Print and shaded views of the part. All mm, measured from the part's lowest x, y and z. Coordinates: 2 decimals unless noted, no trailing zeros. Order: outer loops, then holes, each group sorted by start corner. A loop starts at its lowest first (then second) coordinate and runs counter-clockwise, first axis right, second up.
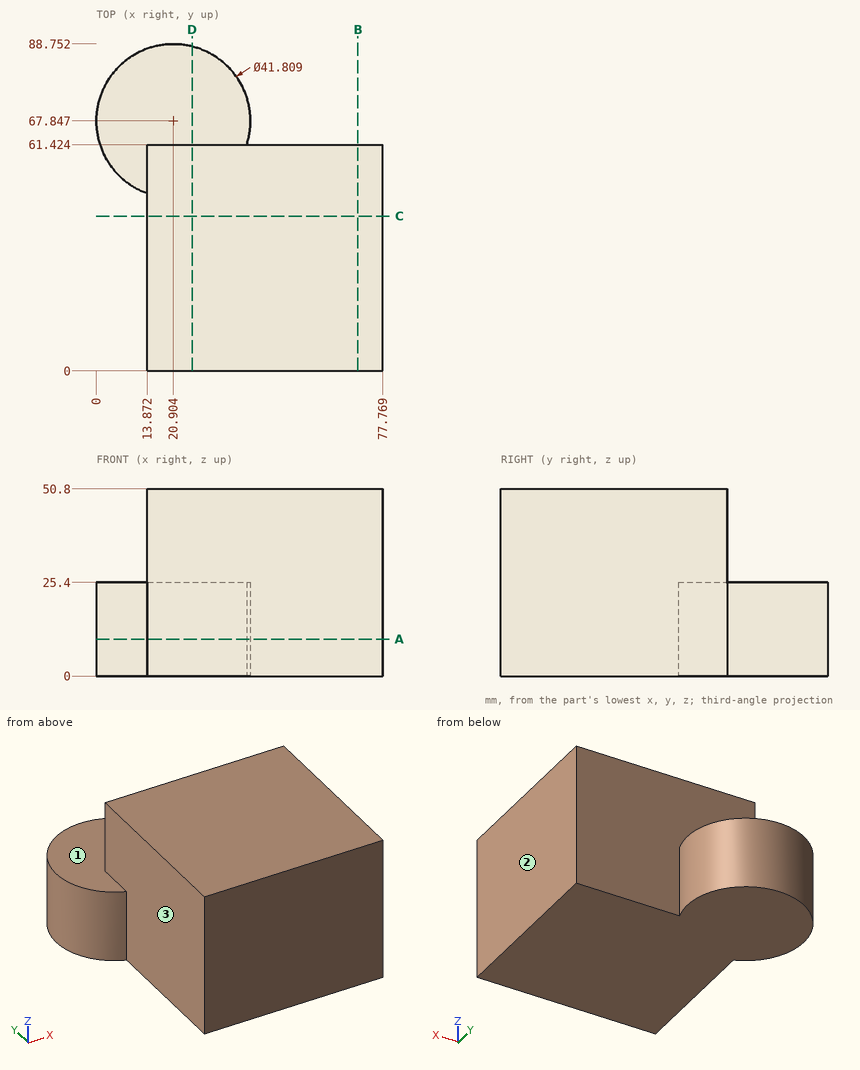
Q1. Cut at A-A, the plane z = 10. List the corners of the cut face in (x, y) (1 decimal).
Established:
outline: (13.9, 0) - (77.8, 0) - (77.8, 61.4) - (40.8, 61.4) arc R20.9 ccw (long way) to (13.9, 48.2) - close
Q2. Cut at D-D, the plane x = 26. List the corners of the cut face in (y, z) (1 decimal).
Established:
outline: (0, 0) - (88.1, 0) - (88.1, 25.4) - (61.4, 25.4) - (61.4, 50.8) - (0, 50.8) - close
Q3. Drop flat-ended pins along their axis: P1, Ø8, axis at x = 8.5, z = 41, coming from the +Y side; P2, Ø15, axis at y = 33, z = 24.5, coming from the -X side. Give the stop position or say it passes through.
Established:
P1: passes through
P2: stops at x = 13.87
Q4. Mould opens along X. For the marked faces 1, 2 and 3 say: pulls with the +X half, pulls with the -X half, needs draft (parallel to the pull), parting line crosses it, or undercut.
Established:
face 1: needs draft
face 2: pulls with the +X half
face 3: pulls with the -X half
Q5. Cut at B-B, the plane x = 71. List the corners of the cut face in (y, z) (1 decimal), plus the area to 3 significant figures.
Established:
outline: (0, 0) - (61.4, 0) - (61.4, 50.8) - (0, 50.8) - close
area: 3,120 mm2
Q6. Probe line 1 (Y direction, x = 63, z = 44.5) (1 decimal); line 2 (Y direction, x = 20, z = 9); line 3 (X direction, y = 26.5, z = 6). List the from-to ranges inside material, lowest first.
Established:
line 1: y = 0 to 61.4
line 2: y = 0 to 88.73
line 3: x = 13.87 to 77.77
Q7. Cut at C-C, the plane y = 42. List the corners of the cut face in (x, z).
Established:
outline: (13.87, 0) - (77.77, 0) - (77.77, 50.8) - (13.87, 50.8) - close
